Here's how the part is built. I have some questions about the finished solid (model axes, mm). Face numbers are marked on the shaded views. A direction names the side the tool comes from. Coordinates: 2 decimals unless noted, no trailing zeros. Order: outer loops, then holes, each group sorted by start corner. A loop starts at its lowest first (then second) coordinate and runs counter-clockwise, first axis right, second up. Notation, with made-up numbers: (31, 54.5) - (79, 54.5) arc R22 ccw to (79, 75.5) - close; hole circle Ø7 at (-38, -1.75). An arc over 180 degrees is marked (long way). Answer in a Markdown table with one row per item. Add a question column.
Item 1: On a 3-axis mill with a long thin cutter (end or side, diameter ignored), from which of +Z, -Z, +X, -X, +Y, -Y can I reach the whole of each face in a straight line? I mean the marked faces 1, 2, 3, 4 and 5. Say none if no direction works.
Item 2: If I drill on line 1 along Y through (x, z) = (35, 10.3) (3 decimals); line 2 along Z through (x, y) = (55, -13.5); line 3 along X through (y, z) = (-16, 7.75), over which ranges is the centre line in solid material (lowest first)? Write a range as from..to.
Item 3: Thinking about a two-plate mould opening in X: for the marked faces 6, 7 and 8, which applies, +X half, -X half, draft (parallel to the pull), parting line (faces both ways), or undercut?
Item 4: I want a section at A-A (y = -3.5). Please give me the cut outline in (x, z), plus the area to 3 significant figures.
Item 5: I want a section at D-D (z = 15). Please give me the cut outline in (x, y) (3 decimals).
Item 6: Will these pins go through, and if not, where does the flat tip stop? pin 1 Ø1.4 at (x, z) = (29, 7.5) entering from -Y; pin 2 Ø6.5 at (x, y) = (8, -10.5) entering from +Z; pin 3 Ø2 at (y, z) = (-15.5, 3) entering from -X.
Item 7: I want a section at C-C (z = 2.5). Count the separate pieces of the cut face and the enclosed holes in it, plus the area to 3 significant figures.
Item 8: I want a section at B-B (x = 9). Please give me the cut outline in (y, z), plus the area to 3 significant figures.
```python
from build123d import *

# Parameters (mm, degrees)
EXTRUSION1_DEPTH             = 2
ESQUISSE2_W                  = 13
ESQUISSE2_H                  = 13
EXTRUSION2_DEPTH             = 11
ESQUISSE7_W                  = 9.4
ESQUISSE7_H                  = 6.8
EXTRUSION7_DEPTH             = 6.1
ESQUISSE8_W                  = 2.8
ESQUISSE8_H                  = 9.5
ESQUISSE8_W_2                = 9.5
ESQUISSE8_H_2                = 2.8
EXTRUSION8_DEPTH             = 11
ESQUISSE6_R                  = 5
EXTRUSION6_DEPTH             = 2
ESQUISSE3_W                  = 6
ESQUISSE3_H                  = 6
EXTRUSION3_DEPTH             = 5
ESQUISSE5_R                  = 2
EXTRUSION5_DEPTH             = 2
ESQUISSE9_W                  = 1.15
ESQUISSE9_H                  = 1.85
EXTRUSION9_DEPTH             = 7.2
EXTRUSION9_DIRECTION_2_REACH = 84.662


with BuildPart() as part:
    # Esquisse1 → Extrusion1 (new body)
    with BuildSketch(Plane.XY):
        Polygon((2.941176471, -27), (25, -27), (25, -42), (45, -42), (45, -27), (67.058823529, -27), (70, -25), (70, -5), (65, 0), (5, 0), (0, -5), (0, -25), align=None)
    extrude(amount=-EXTRUSION1_DEPTH)

    # Esquisse2 → Extrusion2 (add)
    with BuildSketch(Plane.XY):
        with Locations((35, -14.5)):
            Rectangle(ESQUISSE2_W, ESQUISSE2_H)
    extrude(amount=EXTRUSION2_DEPTH)

    # Esquisse7 → Extrusion7 (add)
    with BuildSketch(Plane.XY):
        with Locations((35, -4.6)):
            Rectangle(ESQUISSE7_W, ESQUISSE7_H)
    extrude(amount=EXTRUSION7_DEPTH)

    # Esquisse8 → Extrusion8 (add)
    with BuildSketch(Plane.XY):
        with Locations((27.1, -14.5)):
            Rectangle(ESQUISSE8_W, ESQUISSE8_H)
        with Locations((35, -22.4)):
            Rectangle(ESQUISSE8_W_2, ESQUISSE8_H_2)
    extrude(amount=EXTRUSION8_DEPTH)

    # Esquisse6 → Extrusion6 (cut)
    with BuildSketch(Plane.XY.offset(11)):
        with Locations((35, -14.5)):
            Circle(ESQUISSE6_R)
    extrude(amount=-EXTRUSION6_DEPTH, mode=Mode.SUBTRACT)

    # Esquisse3 → Extrusion3 (add)
    with BuildSketch(Plane.XY):
        with Locations((9, -21)):
            Rectangle(ESQUISSE3_W, ESQUISSE3_H)
        with Locations((9, -10)):
            Rectangle(ESQUISSE3_W, ESQUISSE3_H)
        with Locations((35, -37)):
            Rectangle(ESQUISSE3_W, ESQUISSE3_H)
        with Locations((61, -10)):
            Rectangle(ESQUISSE3_W, ESQUISSE3_H)
        with Locations((61, -21)):
            Rectangle(ESQUISSE3_W, ESQUISSE3_H)
    extrude(amount=EXTRUSION3_DEPTH)

    # Esquisse5 → Extrusion5 (add)
    with BuildSketch(Plane.XY.offset(5)):
        with Locations((9, -10)):
            Circle(ESQUISSE5_R)
        with Locations((9, -21)):
            Circle(ESQUISSE5_R)
        with Locations((61, -21)):
            Circle(ESQUISSE5_R)
        with Locations((61, -10)):
            Circle(ESQUISSE5_R)
        with Locations((35, -37)):
            Circle(ESQUISSE5_R)
    extrude(amount=EXTRUSION5_DEPTH)

    # Esquisse9 → Extrusion9 (add)
    with BuildSketch(Plane.XY.offset(11)):
        with Locations((35, -14.5)):
            Rectangle(ESQUISSE9_W, ESQUISSE9_H)
    extrude(amount=EXTRUSION9_DEPTH)

    # Esquisse9 → Extrusion9 direction 2 (add, up to next)
    with BuildSketch(Plane.XY.offset(11), mode=Mode.PRIVATE) as extrusion9_direction_2_sk1:
        with Locations((35, -14.5)):
            Rectangle(ESQUISSE9_W, ESQUISSE9_H)
    extrusion9_direction_2_tool1 = extrude(extrusion9_direction_2_sk1.sketch, amount=-EXTRUSION9_DIRECTION_2_REACH, mode=Mode.PRIVATE) - part.part
    add(extrusion9_direction_2_tool1.solids().sort_by_distance((35, -14.5, 11))[0])


solid = part.part
```
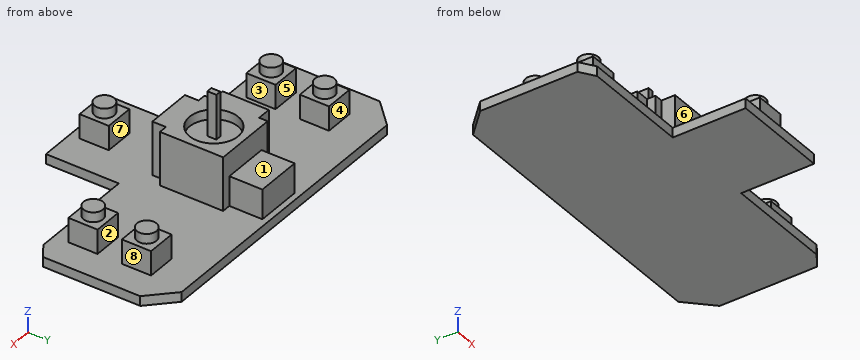
Values follow:
| question | item | result |
|---|---|---|
| 1 | face 1 | +Z, +X, -X, +Y |
| 1 | face 2 | +Z, +X |
| 1 | face 3 | +Z, +Y, -Y |
| 1 | face 4 | +Z, -X, +Y |
| 1 | face 5 | +Z, -X |
| 2 | line 1 | y = -23.8..-19.5, -15.425..-13.575, -9.5..-8 |
| 2 | line 2 | z = -2..0 |
| 2 | line 3 | x = 25.7..41.5 |
| 3 | face 6 | undercut |
| 3 | face 7 | draft |
| 3 | face 8 | +X half |
| 4 | outline | (1.5, -2) - (68.5, -2) - (68.5, 0) - (39.7, 0) - (39.7, 6.1) - (30.3, 6.1) - (30.3, 0) - (1.5, 0) - close |
| 4 | area | 191 mm^2 |
| 5 | outline | (34.425, -15.425) - (35.575, -15.425) - (35.575, -13.575) - (34.425, -13.575) - close |
| 6 | pin 1 | stops at y = -21 |
| 6 | pin 2 | stops at z = 7 |
| 6 | pin 3 | stops at x = 25.7 |
| 7 | separate pieces | 6 |
| 7 | enclosed holes | 0 |
| 7 | area | 466 mm^2 |
| 8 | outline | (-27, -2) - (0, -2) - (0, 0) - (-7, 0) - (-7, 5) - (-8, 5) - (-8, 7) - (-12, 7) - (-12, 5) - (-13, 5) - (-13, 0) - (-18, 0) - (-18, 5) - (-19, 5) - (-19, 7) - (-23, 7) - (-23, 5) - (-24, 5) - (-24, 0) - (-27, 0) - close |
| 8 | area | 130 mm^2 |
